```python
from build123d import *

# Parameters (mm, degrees)
SKETCH2_W               = 40
SKETCH2_H               = 35
BOSS_EXTRUDE1_DEPTH     = 5
SKETCH4_R               = 4.75
BOSS_EXTRUDE2_DEPTH     = 8
SKETCH6_OUTSIDE_W       = 53.224
SKETCH6_OUTSIDE_H       = 48.224
CUT_EXTRUDE2_DEPTH      = 20
CUT_EXTRUDE2_DEPTH_BACK = 20
M6X1_0_TAPPED_HOLE1_D   = 5


with BuildPart() as part:
    # Sketch2 → Boss-Extrude1 (new body)
    with BuildSketch(Plane.XY):
        with Locations((20, 17.5)):
            Rectangle(SKETCH2_W, SKETCH2_H)
    extrude(amount=BOSS_EXTRUDE1_DEPTH)

    # Sketch4 → Boss-Extrude2 (add)
    with BuildSketch(Plane.XY.offset(5)):
        with Locations((25.885379028, 17.5)):
            Circle(SKETCH4_R)
    extrude(amount=BOSS_EXTRUDE2_DEPTH)

    # Mirror4: part across plane


with BuildPart() as part_1:
    add(part.part)
    add(part.part.mirror(Plane.XY.offset(9)))

    # Sketch6 outside → Cut-Extrude2 (cut, two sides)
    with BuildSketch(Plane.XY.offset(5)) as cut_extrude2_sk:
        with Locations((20, 17.5)):
            Rectangle(SKETCH6_OUTSIDE_W, SKETCH6_OUTSIDE_H)
        with BuildLine():
            Line((25.86267887, 31.77132519), (0, 31.77132519))
            Line((0, 31.77132519), (0, 3.496682929))
            Line((0, 3.496682929), (25.86267887, 3.496682929))
            ThreePointArc((25.86267887, 3.496682929), (40, 17.63400406), (25.86267887, 31.77132519))
        make_face(mode=Mode.SUBTRACT)
    extrude(amount=CUT_EXTRUDE2_DEPTH, mode=Mode.SUBTRACT)
    extrude(cut_extrude2_sk.sketch, amount=-CUT_EXTRUDE2_DEPTH_BACK, mode=Mode.SUBTRACT)

    # M6x1.0 Tapped Hole1 (through all)
    with Locations(Plane(origin=(0, 0, 0), x_dir=(-1, 0, 0), z_dir=(0, 0, -1))):
        with Locations((-25.885379028, 17.5)):
            Hole(M6X1_0_TAPPED_HOLE1_D / 2)


solid = part_1.part
```
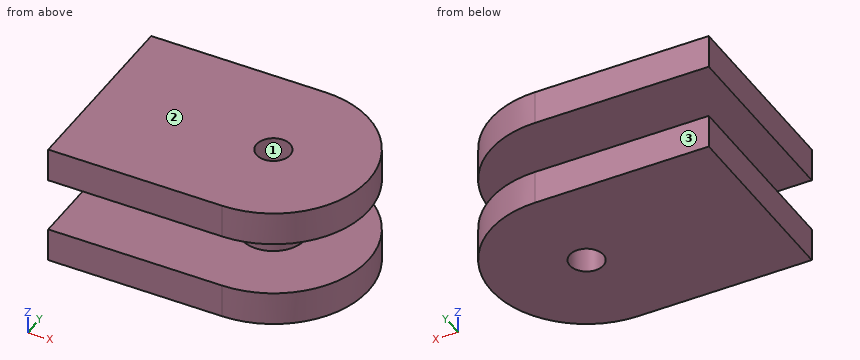
Check sheet for the modelled part. Datum: model origin and axes. Units: mm. Face numbers are marked on the shaded views. Coordinates: 2 decimals unless noted, no trailing zeros. Order: outer loops, then holes, each group sorted by start corner. A loop starts at its lowest first (then second) coordinate and runs counter-clockwise, first axis right, second up. Notation, with made-up numbers: (75.25, -35.5) -> (84.25, -35.5) arc R12 cw to (84.25, -16.5) -> close; hole circle Ø2 at (21, 77). An arc over 180 degrees is marked (long way). Write each question's results on one line, items separated by ' | '. Start each with the question number.
1) Draft check along Y on the marked faces 1, 2 and 3. Enter one of: pulls with the +Y half, pulls with the -Y half, needs draft (parallel to the pull), parting line crosses it, or undercut.
2) Depth check by flat-ended pin: pin 1 (1.5 mm diameter, centred on y = 23.5, z = 8.5, fed in from +X); pin 2 (5 mm diameter, centred on y = 21.5, z = 9.5, fed in from +X); pin 3 (2 mm diameter, centred on y = 14, z = 2.5, fed in from +X). Enter the tip coordinate at first touch or a pass-through.
3) Material ranges on line 1 along Z through (x, y) = (10, 13.75); line 2 along X through (y, z) = (18.75, 13.25); line 3 along Y through (x, z) = (28, 9.25), recorded low to high.
4) Section check A-A (x = 6). Enter the section's corners in (y, z).
5) Section check C-C (y = 29.75). Enter the section's corners in (x, z).
6) Section check D-D (x = 22). Enter the section's corners in (y, z).
Checked values:
1) face 1: undercut | face 2: needs draft | face 3: pulls with the +Y half
2) pin 1: through | pin 2: x = 30.39 | pin 3: x = 39.75
3) line 1: 0 to 5, 13 to 18 | line 2: 0 to 23.72, 28.05 to 39.96 | line 3: 13.25 to 16.17, 18.83 to 21.75
4) outline: (3.5, 0) -> (31.77, 0) -> (31.77, 5) -> (3.5, 5) -> close; (3.5, 13) -> (31.77, 13) -> (31.77, 18) -> (3.5, 18) -> close
5) outline: (0, 0) -> (33.15, 0) -> (33.15, 5) -> (0, 5) -> close; (0, 13) -> (33.15, 13) -> (33.15, 18) -> (0, 18) -> close
6) outline: (3.5, 0) -> (31.77, 0) -> (31.77, 5) -> (20.23, 5) -> (20.23, 13) -> (31.77, 13) -> (31.77, 18) -> (3.5, 18) -> (3.5, 13) -> (14.77, 13) -> (14.77, 5) -> (3.5, 5) -> close
